CAD build for the part. Positions are in the model's coordinates, mm. A direction names the side the tool comes from. Coordinates: 2 decimals unless noted, no trailing zeros. Loops run counter-clockwise (first coordinate to the right, second up) from the corner with the lowest first, then second, coordinate; pieces in that order, holes last. Notation, with made-up numbers: (52, -30) -> (69, -30) arc R28 ccw to (69, -12) -> close; hole circle Ø4 at (-27, -30.75). An arc over 180 degrees is marked (long way). Answer as CSV lines item,"result". Start each with the question number.
```python
from build123d import *

# Parameters (mm, degrees)
BOSS_EXTRUDE1_DEPTH     = 38.1
SKETCH2_3_W             = 12.7
SKETCH2_3_H             = 9.525
SKETCH2_3_W_2           = 8.9535
ARM_RIGHT_DEPTH         = 38.1
CUT_EXTRUDE1_DEPTH      = 48.518879101
CUT_EXTRUDE1_DEPTH_BACK = 48.518879101


with BuildPart() as part:
    # Sketch2 → Boss-Extrude1 (new body)
    with BuildSketch(Plane(origin=(0, 0, 0), x_dir=(1, 0, 0), z_dir=(0, 1, 0))):
        Polygon((-3.6195, 12.699364984), (-3.7465, 0), (-3.7465, -9.525), (3.7465, -9.525), (3.7465, 0), (3.6195, 12.699364984), (1.0795, 12.699364984), (1.2065, 0), (1.2065, -3.556), (-1.2065, -3.556), (-1.2065, 0), (-1.0795, 12.699364984), align=None)
    extrude(amount=BOSS_EXTRUDE1_DEPTH)

    # Sketch2<3> → Arm Right (add)
    with BuildSketch(Plane(origin=(0, 0, 0), x_dir=(1, 0, 0), z_dir=(0, 1, 0))):
        with Locations((19.05, -4.7625)):
            Rectangle(SKETCH2_3_W, SKETCH2_3_H)
        with Locations((8.22325, -4.7625)):
            Rectangle(SKETCH2_3_W_2, SKETCH2_3_H)
    extrude(amount=ARM_RIGHT_DEPTH)

    # Sketch3 → Cut-Extrude1 (cut, two sides: drawn at the far end of the back side and taken through both)
    with BuildSketch(Plane(origin=(0, 0, 0), x_dir=(0, 0, -1), z_dir=(1, 0, 0)).offset(-CUT_EXTRUDE1_DEPTH_BACK)):
        Polygon((-5.715, 0), (-3.556, 0), (-3.429, 31.75), (-5.842, 31.75), align=None)
    extrude(amount=CUT_EXTRUDE1_DEPTH + CUT_EXTRUDE1_DEPTH_BACK, mode=Mode.SUBTRACT)


solid = part.part
```
Q1. Saw through at C-C (x = 21). List the corners of the cut face in (y, z) (3 decimals), and give its area (3 significant figures).
Q2. Two-plate mould, pull along X, no slides. Class faces 1 (the flat face through (11, 31.75, 5)), 2 (the flat face through (-1.206, 19, 2)), 3 (the flat face through (25.4, 19, 6)): pulls with the +X half, pulls with the -X half, needs draft (parallel to the pull), parting line crosses it, or undercut.
Q3. Saw through at D-D (y = 33). List the corners of the cut face in (x, z) (1 decimal), and give its area (3 significant figures).
Q4. Probe probe 1 along Z at (x, y) = (14.75, 31) (3 decimals); probe 2 along Z at (x, y) = (8, 2) (3 decimals); probe 3 along Y at (x, z) = (4.5, 5.5). List the from-to ranges inside material, lowest first. Write a range as from..to.
Q5. Pin check, flat tips, straight feed: pin 1 Ø3 at (x, y) = (15, 29.5) entering from -Z; pin 2 Ø8 at (y, z) = (5, -9.5) entering from -X. Stop position of each tip, or through.
Q6. Which spindle directions (+Z, -Z, +X, -X, +Y, -Y) get a long thin tool onto all of the face, cutting with end or side? Do faces 4 (the flat face through (11, 0, 8)), 5 (the flat face through (1.206, 19, 2)), 6 (the flat face through (15, 19, 0)). Say none if no direction does.
Q7. Saw through at B-B (y = 14). List the corners of the cut face in (x, z) (1 decimal).
Q8. Saw through at A-A (z = 2.5). List the corners of the cut face in (x, y).
Ans:
1,outline,"(0, 0) -> (38.1, 0) -> (38.1, 9.525) -> (0, 9.525) -> (0, 5.715) -> (31.75, 5.842) -> (31.75, 3.429) -> (0, 3.556) -> close"
1,area,"290 mm²"
2,face 1,"needs draft"
2,face 2,"undercut"
2,face 3,"pulls with the +X half"
3,outline,"(-3.7, 0) -> (-3.6, -12.7) -> (-1.1, -12.7) -> (-1.2, 0) -> (-1.2, 3.6) -> (1.2, 3.6) -> (1.2, 0) -> (1.1, -12.7) -> (3.6, -12.7) -> (3.7, 0) -> (25.4, 0) -> (25.4, 9.5) -> (-3.7, 9.5) -> close"
3,area,"334 mm²"
4,probe 1,"z = 0..3.432, 5.839..9.525"
4,probe 2,"z = 0..3.548, 5.723..9.525"
4,probe 3,"y = 31.75..38.1"
5,pin 1,"stops at z = 0"
5,pin 2,"stops at x = -3.69"
6,face 4,"+Z, -Z, +X, -X, -Y"
6,face 5,"+Y, -Y"
6,face 6,"-Z, +X, +Y, -Y"
7,outline,"(-3.7, 0) -> (-3.6, -12.7) -> (-1.1, -12.7) -> (-1.2, 0) -> (-1.2, 3.5) -> (-3.7, 3.5) -> close; (-3.7, 5.8) -> (25.4, 5.8) -> (25.4, 9.5) -> (-3.7, 9.5) -> close; (1.1, -12.7) -> (3.6, -12.7) -> (3.7, 0) -> (25.4, 0) -> (25.4, 3.5) -> (1.2, 3.5) -> (1.2, 0) -> close"
8,outline,"(-3.75, 0) -> (-1.21, 0) -> (-1.21, 38.1) -> (-3.75, 38.1) -> close; (1.21, 0) -> (25.4, 0) -> (25.4, 38.1) -> (1.21, 38.1) -> close"
